Print and shaded views of the part. All mm, measured from the part's lowest x, y and z. Round coordinates to 2 decimals unless told otherwise and drop trailing zeros. Loops run counter-clockwise (first coordinate to the right, second up) from the corner with the lowest first, then second, coordinate; pieces in that order, holes last. Notation, with made-up numbers: (-7, -20) - (40, -20) arc R35 ccw to (40, 13) - close; hole circle Ø8 at (14, -39). An arc over 180 degrees is marked (long way). Use one line per item in the form item = value.
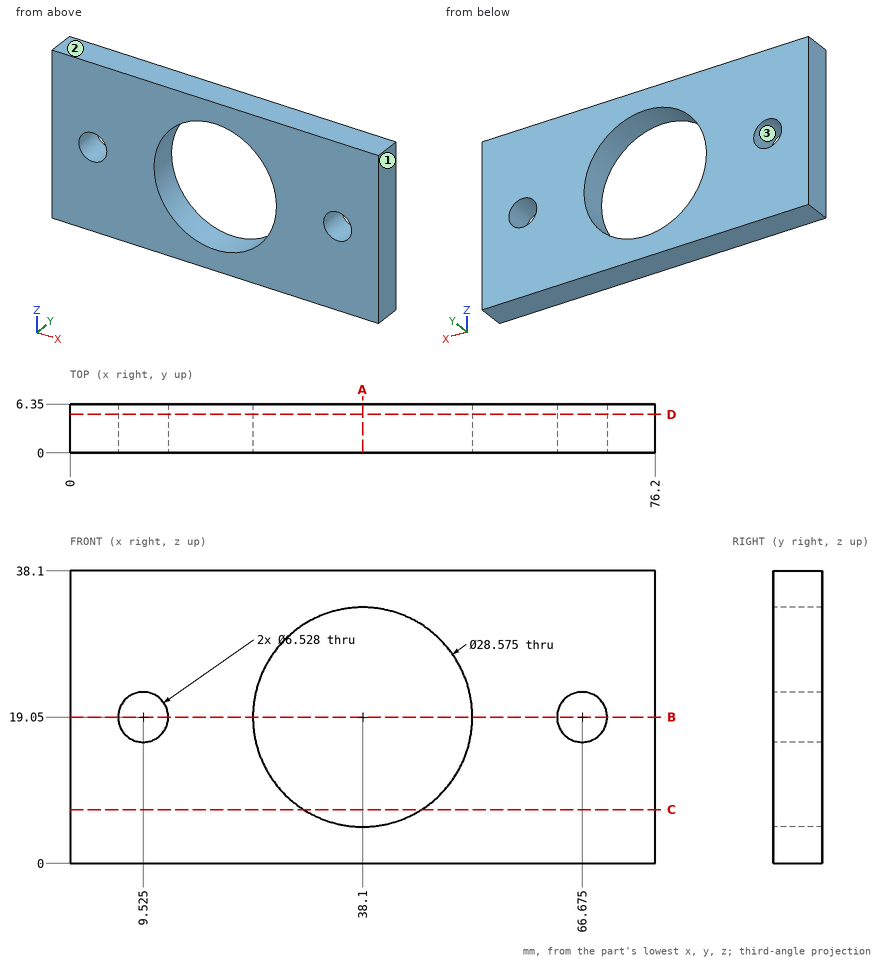
1. Cut at A-A, the plane x = 38.1. Give the cut face in (y, z).
Geometry check:
outline = (0, 0) - (6.35, 0) - (6.35, 4.76) - (0, 4.76) - close; (0, 33.34) - (6.35, 33.34) - (6.35, 38.1) - (0, 38.1) - close
2. Cut at B-B, the plane z = 19.05. Give the cut face in (x, y).
Geometry check:
outline = (0, 0) - (6.26, 0) - (6.26, 6.35) - (0, 6.35) - close; (12.79, 0) - (23.81, 0) - (23.81, 6.35) - (12.79, 6.35) - close; (52.39, 0) - (63.41, 0) - (63.41, 6.35) - (52.39, 6.35) - close; (69.94, 0) - (76.2, 0) - (76.2, 6.35) - (69.94, 6.35) - close
3. Cut at C-C, the plane z = 7. Give the cut face in (x, y).
Geometry check:
outline = (0, 0) - (30.42, 0) - (30.42, 6.35) - (0, 6.35) - close; (45.78, 0) - (76.2, 0) - (76.2, 6.35) - (45.78, 6.35) - close
4. Pull direction Z, two halves, no side cores. Call the marked faces 1, 2 and 3: +Z half, -Z half, draft (parallel to the pull), parting line (faces both ways), or undercut.
Geometry check:
face_1 = draft
face_2 = +Z half
face_3 = undercut
5. Wall check: probe 1 along X at (y, z) = (3.75, 19.05); probe 2 along X at (y, z) = (6, 20); probe 3 along Z at (x, y) = (38.1, 2.75). Give the ranges that are in metal, low to high.
Geometry check:
probe_1 = 0 to 6.26, 12.79 to 23.81, 52.39 to 63.41, 69.94 to 76.2
probe_2 = 0 to 6.4, 12.65 to 23.84, 52.36 to 63.55, 69.8 to 76.2
probe_3 = 0 to 4.76, 33.34 to 38.1
6. Flat gauge pin, fed straight in: pin 1 (4 mm diameter, centred on x = 66.675, z = 19.05, fed in from -Y). Where does the tip first touch, or does it go through?
Geometry check:
pin_1 = through
7. Cut at D-D, the plane y = 5. Give the number of separate pieces and of enclosed holes in the cut face, plus the area to 4 significant figures.
Geometry check:
separate_pieces = 1
enclosed_holes = 3
area = 2,195 mm^2
